Could you check a few things on this model? Use its own coordinates, in mm. A direction names the side the tool comes from. Round coordinates to 2 decimals unless told otherwise and drop trailing zeros. Loops run counter-clockwise (first coordinate to the right, second up) from the corner with the lowest first, then second, coordinate; pieces in that order, holes last.
from build123d import *

# Parameters (mm, degrees)
EXTRUDE_1_DEPTH       = 244
EXTRUDE_3_DEPTH       = 244
PATTERN_CURVE_1_COUNT = 11
PATTERN_CURVE_1_PITCH = 10
SKETCH_3_R            = 2.25
CUT_EXTRUDE_1_DEPTH   = 6
SKETCH_4_R            = 2.6
SKETCH_4_R_2          = 1.6
CUT_EXTRUDE_2_DEPTH   = 6
SKETCH_5_R            = 2.1
SKETCH_5_R_2          = 1.6
CUT_EXTRUDE_3_DEPTH   = 6


with BuildPart() as part:
    # Эскиз1 → Вытянуть1 (new body)
    with BuildSketch(Plane.XY):
        with BuildLine():
            Line((0, 40), (1.528979332, 40))
            ThreePointArc((1.528979332, 40), (2.225614441, 39.717425624), (2.528547087, 39.029399052))
            Line((2.528547087, 39.029399052), (3.5, 6))
            Line((3.5, 6), (118.5, 6))
            Line((118.5, 6), (119.471452913, 39.029399052))
            ThreePointArc((119.471452913, 39.029399052), (119.774385559, 39.717425624), (120.471020668, 40))
            Line((120.471020668, 40), (122, 40))
            Line((122, 40), (122, 0))
            Line((122, 0), (0, 0))
            Line((0, 0), (0, 40))
        make_face()
    extrude(amount=EXTRUDE_1_DEPTH)

    # Эскиз2 → Вытянуть3 (add)
    with BuildSketch(Plane.XY.offset(244)):
        with BuildLine():
            Line((10.5, 39.5), (9.25, 6))
            Line((9.25, 6), (12.75, 6))
            Line((12.75, 6), (11.5, 39.5))
            ThreePointArc((11.5, 39.5), (11, 40), (10.5, 39.5))
        make_face()
    extrude_3 = extrude(amount=-EXTRUDE_3_DEPTH)

    # Кривая1: Вытянуть3 ×11
    with Locations(*[(i * PATTERN_CURVE_1_PITCH, 0, 0) for i in range(1, PATTERN_CURVE_1_COUNT)]):
        add(extrude_3)

    # Эскиз3 → Вырез-Вытянуть1 (cut)
    with BuildSketch(Plane.XZ):
        with Locations((26, 236)):
            Circle(SKETCH_3_R)
        with Locations((96, 236)):
            Circle(SKETCH_3_R)
        with Locations(Location((96, 8, 0), (0, 0, 180))):
            Circle(SKETCH_3_R)
        with Locations(Location((26, 8, 0), (0, 0, 180))):
            Circle(SKETCH_3_R)
    extrude(amount=-CUT_EXTRUDE_1_DEPTH, mode=Mode.SUBTRACT)

    # Эскиз4 → Вырез-Вытянуть2 (cut)
    with BuildSketch(Plane(origin=(-5.723570629, 0, -26.359021189), x_dir=(1, 0, 0), z_dir=(0, -1, 0))):
        with Locations((94.223570629, 89.359021189)):
            Circle(SKETCH_4_R)
        with Locations((67.723570629, 187.359021189)):
            Circle(SKETCH_4_R_2)
        with Locations((67.723570629, 52.359021189)):
            Circle(SKETCH_4_R_2)
        with Locations((107.973570629, 183.759021189)):
            Circle(SKETCH_4_R_2)
        with Locations((107.973570629, 99.959021189)):
            Circle(SKETCH_4_R_2)
    extrude(amount=-CUT_EXTRUDE_2_DEPTH, mode=Mode.SUBTRACT)

    # Эскиз5 → Вырез-Вытянуть3 (cut)
    with BuildSketch(Plane(origin=(128.324191418, 0, 423.775874855), x_dir=(-1, 0, 0), z_dir=(0, -1, 0))):
        with Locations(Location((89.324191418, 279.775874855, 0), (0, 0, 180))):
            Circle(SKETCH_5_R)
        with Locations((21.324191418, 239.775874855)):
            Circle(SKETCH_5_R_2)
        with Locations((81.324191418, 239.775874855)):
            Circle(SKETCH_5_R_2)
        with Locations(Location((81.324191418, 204.775874855, 0), (0, 0, 180))):
            Circle(SKETCH_5_R_2)
        with Locations(Location((21.324191418, 204.775874855, 0), (0, 0, 180))):
            Circle(SKETCH_5_R_2)
    extrude(amount=-CUT_EXTRUDE_3_DEPTH, mode=Mode.SUBTRACT)


solid = part.part
Item 1: If we section it at A-A, the plane z = 8: Count the separate pieces of the cut face and the enclosed holes in it, then the cut area to 3 significant figures.
Results list:
separate pieces: 3
enclosed holes: 0
area: 1,720 mm2
Item 2: If I drill on line 1 along X through (y, z) = (3, 219); line 2 along Z through (x, y) = (62, 1.55); line 3 along Z through (x, y) = (26, 2), over which ranges is the centre line in solid material (lowest first)?
Results list:
line 1: x = 0 to 45.4, 48.6 to 105.4, 108.6 to 122
line 2: z = 0 to 24.4, 27.6 to 159.4, 162.6 to 244
line 3: z = 0 to 5.75, 10.25 to 233.75, 238.25 to 244
Item 3: Will these pins go through, and if not, where does the flat tip stop? pin 1 (7 mm diameter, centred on x = 27.5, z = 166, fed in from +Y); pin 2 (1.9 mm diameter, centred on x = 62, z = 161.5, fed in from -Y); pin 3 (2 mm diameter, centred on x = 98, z = 136, fed in from +Y).
Results list:
pin 1: stops at y = 40
pin 2: stops at y = 6
pin 3: stops at y = 6
Item 4: For faces 1 (the flat face through (86, 6, 120)), 2 (the cylindrical face through (23.854, 2.958, 7.324)), which set-ups out of +Z, -Z, +X, -X, +Y, -Y let a thin tool reach every point of the face, with its end or its side?
Results list:
face 1: +Z, -Z, +Y
face 2: +Y, -Y
Item 5: We'd pull the mould along X, two halves only. Please class faces 3 (the flat face through (62, 0, 120)), 4 (the flat face through (46, 6, 120)), 5 (the flat face through (32.134, 22.516, 123.708)): released by +X, released by -X, zero draft, split by the parting line, or undercut.
Results list:
face 3: zero draft
face 4: undercut
face 5: undercut
Item 6: If we section it at C-C, the plane x = 55: Please give me the cut outline in (y, z), then the cut area to 3 significant figures.
Results list:
outline: (0, 0) - (6, 0) - (6, 244) - (0, 244) - close
area: 1,460 mm2
